Job drawing, mm, ordinate dimensions from the low corner. One solid piece. A direction names the side the tool comes from. Round coordinates to 2 decimals unless told otherwise and drop trailing zeros. Write each loop counter-clockwise with the first axis right and the second up, starting at its lowest first coordinate (ties: lowest second). Pieces come first, ordered by that corner, then holes.
1) Which spindle directions (+Z, -Z, +X, -X, +Y, -Y) get a long thin tool onto all of the face, cutting with end or side? Do the marked faces 1, 2 and 3. Say none if no direction does.
2) Saw through at B-B on x = 24. Write the cut outline in (y, z).
3) Drill centre lines: L1, parallel to Z at x = 24, y = 1.8; L2, parallel to Y at x = 3.75, z = 19.5; L3, parallel to Y at x = 18.25, z = 20. Where is each one in solid material? Low to high.
4) Saw through at A-A on z = 9. Write the cut outline in (x, y).
5) Saw through at D-D on y = 38. Write the cut outline in (x, z).
6) Flat gauge pins, fed straight in: pin 1 (1 mm diameter, centred on x = 22.5, z = 4.5, fed in from +Y); pin 2 (8 mm diameter, centred on x = 5.5, z = 15, fed in from +Y); pin 3 (20 mm diameter, centred on y = 38, z = 20, fed in from -X). Where does each tip first touch, or does it go through?
7) Saw through at C-C on z = 16.5. Write the cut outline in (x, y).
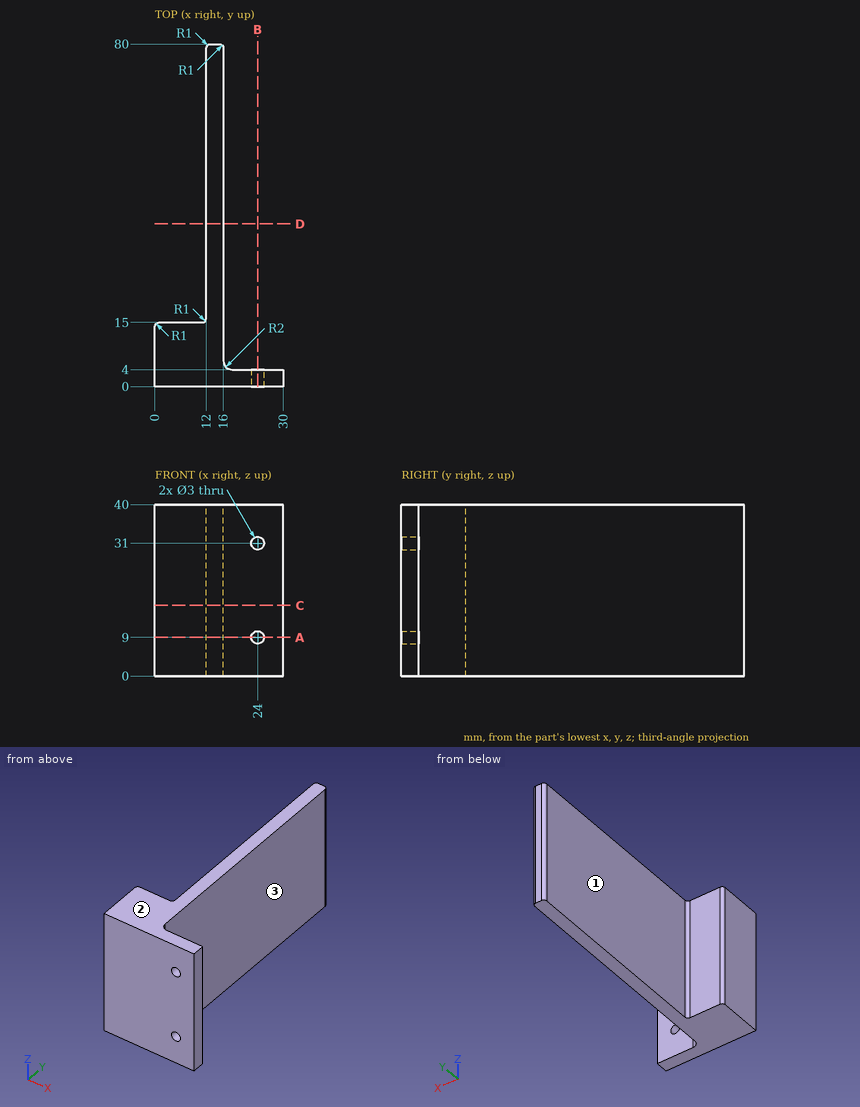
Completed:
1. face 1: +Z, -Z, -X, +Y
1. face 2: +Z, +X, -X, +Y, -Y
1. face 3: +Z, -Z, +X, +Y
2. outline: (0, 0) - (4, 0) - (4, 7.5) - (0, 7.5) - close; (0, 10.5) - (4, 10.5) - (4, 29.5) - (0, 29.5) - close; (0, 32.5) - (4, 32.5) - (4, 40) - (0, 40) - close
3. L1: z = 0 to 7.5, 10.5 to 29.5, 32.5 to 40
3. L2: y = 0 to 15
3. L3: y = 0 to 4
4. outline: (0, 0) - (22.5, 0) - (22.5, 4) - (18, 4) arc R2 cw to (16, 6) - (16, 79) arc R1 ccw to (15, 80) - (13, 80) arc R1 ccw to (12, 79) - (12, 16) arc R1 cw to (11, 15) - (1, 15) arc R1 ccw to (0, 14) - close; (25.5, 0) - (30, 0) - (30, 4) - (25.5, 4) - close
5. outline: (12, 0) - (16, 0) - (16, 40) - (12, 40) - close
6. pin 1: stops at y = 4
6. pin 2: stops at y = 15
6. pin 3: stops at x = 12
7. outline: (0, 0) - (30, 0) - (30, 4) - (18, 4) arc R2 cw to (16, 6) - (16, 79) arc R1 ccw to (15, 80) - (13, 80) arc R1 ccw to (12, 79) - (12, 16) arc R1 cw to (11, 15) - (1, 15) arc R1 ccw to (0, 14) - close
